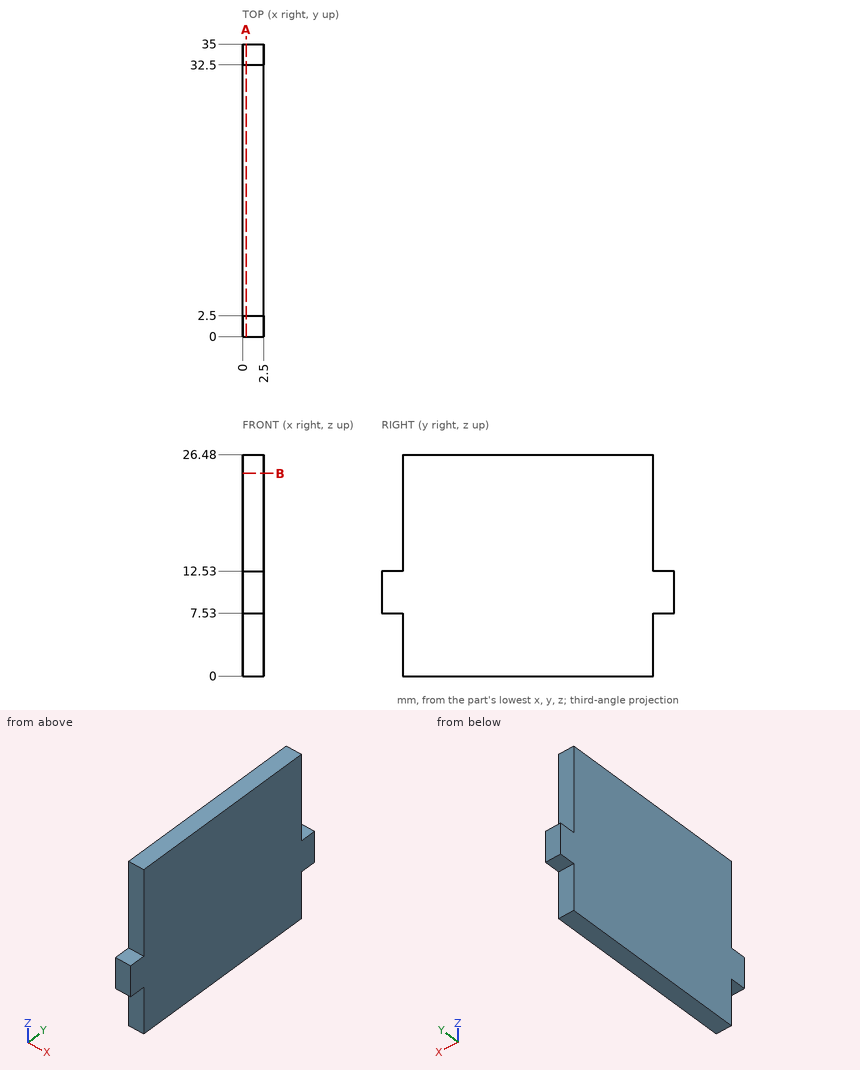
Here's the drawing with two shaded views (mm, measured from the low corner). I have some questions. Coordinates: 2 decimals unless noted, no trailing zeros. Loops run counter-clockwise (first coordinate to the right, second up) from the corner with the lowest first, then second, coordinate; pieces in that order, holes last. Notation, with made-up numbers: (-16.75, 2.25) -> (12.25, 2.25) arc R35 cw to (12.25, 41.25) -> close; hole circle Ø10 at (-6, 6.25). An arc over 180 degrees is marked (long way). Put each result on its own line as item: value. Start each with the question number.
Q1. I want a section at A-A (x = 0.4). Write out the boundary of the cut face in (y, z), plus the area to 3 significant figures.
Q2. If I drill on line 1 (Y direction, x = 1.95, z = 22); line 2 (Z direction, x = 1.3, y = 33), over which ranges is the centre line in solid material (lowest first)? Write a range as [from, to].
Q3. I'm going to push flat-ended pins straight in: P1, Ø0.8, axis at x = 1.5, z = 16, coming from the +Y side; P2, Ø0.8, axis at x = 1.5, z = 5.5, coming from the -Y side; P3, Ø1.2, axis at x = 0.5, y = 1.5, coming from the +Z side. Where does each tip first touch, or does it pass through?
Q4. I want a section at B-B (z = 24.25). Write out the boundary of the cut face in (x, y), plus the area to 3 significant figures.
Taken from the geometry:
1. outline: (0, 7.53) -> (2.5, 7.53) -> (2.5, 0) -> (32.5, 0) -> (32.5, 7.53) -> (35, 7.53) -> (35, 12.53) -> (32.5, 12.53) -> (32.5, 26.48) -> (2.5, 26.48) -> (2.5, 12.53) -> (0, 12.53) -> close
1. area: 819 mm2
2. line 1: y = [2.5, 32.5]
2. line 2: z = [7.53, 12.53]
3. P1: stops at y = 32.5
3. P2: stops at y = 2.5
3. P3: stops at z = 12.53
4. outline: (0, 2.5) -> (2.5, 2.5) -> (2.5, 32.5) -> (0, 32.5) -> close
4. area: 75.0 mm2
